Autodesk Fusion 360 part; units mm, degrees
sketch "Sketch1" plane through (0, 0, 0) normal (0, 0, 1) x (1, 0, 0)
  line L0 (15, 0) -> (65, 0)
  line L1 (65, 30) -> (15, 30)
  arc A0 (15, 30) -> (0, 15) centre (15, 15) ccw
  arc A1 (0, 15) -> (15, 0) centre (15, 15) ccw
  arc A2 (80, 15) -> (65, 30) centre (65, 15) ccw
  arc A3 (65, 0) -> (80, 15) centre (65, 15) ccw
  line L2 (15, 15) -> (65, 15) construction
  line L3 (15, 15) -> (15, 27.5) construction
  line L4 (65, 15) -> (65, 27.5) construction
  line L5 (15, 27.5) -> (40, 27.5) construction
  circle A4 centre (15, 27.5) radius 1.5
  circle A5 centre (40, 27.5) radius 1.5
  circle A6 centre (65, 27.5) radius 1.5
  circle A7 centre (15, 2.5) radius 1.5
  circle A8 centre (40, 2.5) radius 1.5
  circle A9 centre (65, 2.5) radius 1.5
  circle A10 centre (65, 15) radius 2.5
  circle A11 centre (15, 15) radius 2.5
  point P0 (80, 0)
  point P1 (0, 30)
  dimension "d1" = 80
  dimension "d2" = 30
  dimension "d3" = 15
  dimension "d4" = 15
  dimension "d5" = 15
  dimension "d6" = 15
  dimension "d7" = 12.5
  dimension "d8" = 12.5
  dimension "d9" = 25
  dimension "d11" = 3
  dimension "d12" = 3
  dimension "d13" = 3
  dimension "d22" = 5
  dimension "d23" = 5
extrude "Extrude1" add sketch "Sketch1" along normal blind 16 contours L0 L1 A0 A1 A2 A3 | A10 | A11
shell "Shell1" thickness 2 removed faces 1 at (23.6999, 18.8266, 16)
hole "Hole1" at (65, 27.5, 0) at (40, 27.5, 0) at (15, 27.5, 0) at (15, 2.5, 0) at (40, 2.5, 0) at (65, 2.5, 0) direction (0, 0, -1) diameter 4 depth 1 tip angle 180 countersink diameter 4.4 countersink angle 90
extrude "Extrude2" add sketch "Sketch1" against normal blind 4 draft -15 contours A10 | A11
equation "d23 = d22"
Here's how the part is built. I have some questions about the finished solid (model axes, mm). Give positions to 0.01 mm unless a question says otherwise; leave off trailing zeros. Loops run counter-clockwise (first coordinate to the right, second up) from the corner with the lowest first, then second, coordinate; pieces in that order, holes last. Notation, with made-up numbers: (29.5, 9.25) -> (73.5, 9.25) arc R23 ccw to (73.5, 43.25) -> close; hole circle Ø7 at (48, 35). An arc over 180 degrees is marked (long way). One line per item, written item: value.
Q1. If I drill on line 1 along Y through (x, z) = (40, 5); line 2 along X through (y, z) = (28.25, 6.5); line 3 along Z through (x, y) = (23.5, 11.25), over which ranges is the centre line in solid material (lowest first)?
Answers follow:
line 1: 0 to 1, 4 to 26, 29 to 30
line 2: 7.97 to 13.7, 16.3 to 38.7, 41.3 to 63.7, 66.3 to 72.03
line 3: 0 to 16
Q2. We'd pull the mould along X, two halves only. Please class faces 1 (the face through (40, 0, 8)), 2 (the face through (15.855, 13.357, -2.416)), 3 (the face through (80, 15, 8)): pulls with the +X half, pulls with the -X half, needs draft (parallel to the pull), parting line crosses it, or undercut.
Answers follow:
face 1: needs draft
face 2: undercut
face 3: pulls with the +X half
Q3. Suppose I cut it at D-D on y = 27.5. Please give me the cut outline in (x, z), then the cut area to 3 significant figures.
Answers follow:
outline: (6.71, 0) -> (13.5, 0) -> (13.5, 16) -> (6.71, 16) -> close; (16.5, 0) -> (38.5, 0) -> (38.5, 16) -> (16.5, 16) -> close; (41.5, 0) -> (63.5, 0) -> (63.5, 16) -> (41.5, 16) -> close; (66.5, 0) -> (73.29, 0) -> (73.29, 16) -> (66.5, 16) -> close
area: 921 mm^2
Q4. Suppose I cut it at B-B on y = 15. Please give me the cut outline in (x, z), then the cut area to 3 significant figures.
Answers follow:
outline: (0, 0) -> (12.5, 0) -> (13.57, -4) -> (16.43, -4) -> (17.5, 0) -> (62.5, 0) -> (63.57, -4) -> (66.43, -4) -> (67.5, 0) -> (80, 0) -> (80, 16) -> (0, 16) -> close
area: 1,310 mm^2
Q5. Suppose I cut it at C-C on x = 40. Please give me the cut outline in (y, z).
Answers follow:
outline: (0, 0) -> (1, 0) -> (1, 16) -> (0, 16) -> close; (4, 0) -> (26, 0) -> (26, 16) -> (4, 16) -> close; (29, 0) -> (30, 0) -> (30, 16) -> (29, 16) -> close
Q6. I'm going to push flat-ended pins straight in: pin 1 Ø3 at (y, z) = (21, 0) entering from -X; pin 2 Ø1.8 at (x, y) = (40, 2.5) entering from +Z; pin 3 Ø4 at (x, y) = (15, 2.5) entering from -Z; pin 4 Ø5 at (x, z) = (8.5, 7.5) entering from -Y. Where does each tip first touch, or does it pass through?
Answers follow:
pin 1: x = 0.69
pin 2: through
pin 3: z = 0
pin 4: y = 0.54
Q7. Suppose I cut it at A-A on z = 6.25. Please give me the cut outline in (x, y), then the cut area to 3 significant figures.
Answers follow:
outline: (15, 0) -> (65, 0) arc R15 ccw to (65, 30) -> (15, 30) arc R15 ccw to start; hole circle Ø3 at (15, 2.5); hole circle Ø3 at (15, 27.5); hole circle Ø3 at (40, 2.5); hole circle Ø3 at (40, 27.5); hole circle Ø3 at (65, 2.5); hole circle Ø3 at (65, 27.5)
area: 2,160 mm^2
